Part model, mm, in its own coordinate system. Face numbers are marked on the shaded views. A direction names the side the tool comes from. Coordinates: 2 decimals unless noted, no trailing zeros. Write each loop counter-clockwise with the first axis right and the second up, starting at its lowest first coordinate (ties: lowest second). Pieces come first, ordered by that corner, then holes. Notation, with made-up numbers: (-39, -35.5) -> (-12, -35.5) arc R3 ccw to (-12, -30.5) -> close; hole circle Ø8 at (18.25, -38.75). An arc over 180 degrees is marked (long way). Write item = value, one per line.
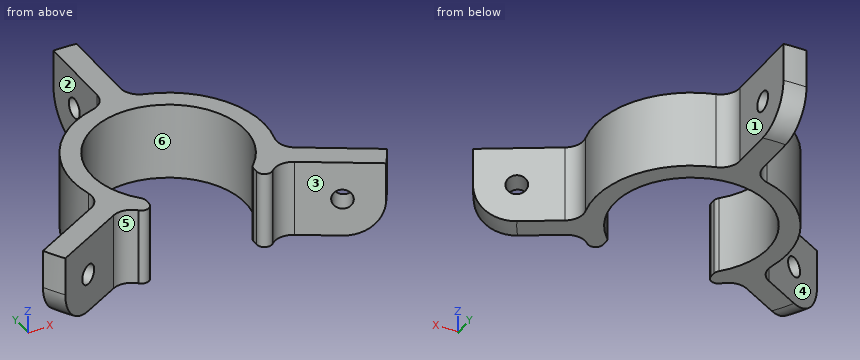
from build123d import *

# Parameters (mm, degrees)
SKETCH_R              = 50
SKETCH_R_2            = 20
PAD_DEPTH             = 20
POCKET_DEPTH          = 305.658137
POLARPATTERN_COUNT    = 3
SKETCH002_W           = 28
SKETCH002_H           = 22.742476
POCKET001_DEPTH       = 20.001
SKETCH003_R           = 2.6
POCKET002_DEPTH       = 287.850495
POLARPATTERN001_COUNT = 3
FILLET_R              = 2
FILLET001_R           = 5
FILLET002_R           = 10


with BuildPart() as part:
    # Sketch → Pad (new body)
    with BuildSketch(Plane.XY):
        Circle(SKETCH_R)
        Circle(SKETCH_R_2, mode=Mode.SUBTRACT)
    extrude(amount=PAD_DEPTH)

    # Sketch001 (on Face4 of Pad) → Pocket (cut, through all)
    with BuildSketch(Plane.XY.offset(20)):
        with BuildLine():
            ThreePointArc((22.994185, -9.811597), (21.650635, 12.5), (3, 24.819347))
            Line((3, 55.952225), (3, 24.819347))
            ThreePointArc((49.956048, -25.378036), (48.525649, 28.016297), (3, 55.952225))
            Line((22.994185, -9.811597), (49.956048, -25.378036))
        make_face()
    pocket = extrude(amount=-POCKET_DEPTH, mode=Mode.SUBTRACT)

    # PolarPattern: Pocket ×3 about axis
    polarpattern_axis = Axis((0, 0, 20), (0, 0, 1))
    for i in range(1, POLARPATTERN_COUNT):
        add(pocket.rotate(polarpattern_axis, i * 360 / POLARPATTERN_COUNT), mode=Mode.SUBTRACT)

    # Sketch002 (on Face4 of PolarPattern) → Pocket001 (cut, through all)
    with BuildSketch(Plane.XY.offset(20)):
        with Locations((0, -23.477223)):
            Rectangle(SKETCH002_W, SKETCH002_H)
    extrude(amount=-POCKET001_DEPTH, mode=Mode.SUBTRACT)

    # Sketch003 (on Face5 of Pocket001) → Pocket002 (cut, through all)
    with BuildSketch(Plane.YZ.offset(3)):
        with Locations((39.909919, 10)):
            Circle(SKETCH003_R)
    pocket002 = extrude(amount=-POCKET002_DEPTH, mode=Mode.SUBTRACT)

    # PolarPattern001: Pocket002 ×3 about axis
    polarpattern001_axis = Axis((0, 0, 0), (0, 0, 1))
    for i in range(1, POLARPATTERN001_COUNT):
        add(pocket002.rotate(polarpattern001_axis, i * 360 / POLARPATTERN001_COUNT), mode=Mode.SUBTRACT)

    # Fillet
    fillet_edges = [part.edges().sort_by_distance(p)[0] for p in [
        (-14, -20.712315, 10),
        (14, -20.712315, 10),
        (14, -14.282857, 10),
        (-14, -14.282857, 10),
    ]]
    fillet(fillet_edges, radius=FILLET_R)

    # Fillet001
    fillet001_edges = [part.edges().sort_by_distance(p)[0] for p in [
        (3, 24.819347, 10),
        (22.994185, -9.811597, 10),
        (-3, 24.819347, 10),
        (-22.994185, -9.811597, 10),
        (-19.994185, -15.00775, 10),
        (19.994185, -15.00775, 10),
    ]]
    fillet(fillet001_edges, radius=FILLET001_R)

    # Fillet002
    fillet002_edges = [part.edges().sort_by_distance(p)[0] for p in [
        (43.30127, -25, 0),
        (-43.30127, -25, 0),
        (0, 50, 0),
    ]]
    fillet(fillet002_edges, radius=FILLET002_R)


solid = part.part
Q1. Pin check, flat tips, straight feed: pin 1 (10 mm diameter, centred on x = 26.5, z = 7, fed in from +Y); pin 2 (10 mm diameter, centred on x = -17, z = 11, fed in from +Y); pin 3 (5 mm diameter, centred on x = -2, z = 13.5, fed in from -Y). Stop position of each tip, or through.
Model answer:
pin_1 = 12.76
pin_2 = 21.93
pin_3 = 19.49
Q2. Saw through at D-D on z = 3.5. Give the cut face in (x, y), and give its area (3 significant figures).
Model answer:
outline = (-42.64, -21.15) arc R47.6 ccw to (-39.64, -26.35) -> (-23.54, -17.05) arc R5 cw to (-17.53, -17.82) arc R25 ccw to (-17.39, -17.96) arc R2 ccw to (-14, -16.52) -> (-14, -15.1) arc R2 ccw to (-14.55, -13.73) arc R20 cw (long way) to (14.55, -13.73) arc R2 ccw to (14, -15.1) -> (14, -16.52) arc R2 ccw to (17.39, -17.96) arc R25 ccw to (17.53, -17.82) arc R5 cw to (23.54, -17.05) -> (39.64, -26.35) arc R47.6 ccw to (42.64, -21.15) -> (26.54, -11.86) arc R5 cw to (24.2, -6.27) arc R25 ccw to (6.67, 24.09) arc R5 cw to (3, 28.91) -> (3, 47.5) arc R47.6 ccw to (-3, 47.5) -> (-3, 28.91) arc R5 cw to (-6.67, 24.09) arc R25 ccw to (-24.2, -6.27) arc R5 cw to (-26.54, -11.86) -> close
area = 973 mm²
Q3. Saw through at C-C on x = 0. Give the cut face in (y, z).
Model answer:
outline = (20, 0) -> (40, 0) arc R10 ccw to (50, 10) -> (50, 20) -> (20, 20) -> close; hole circle Ø5.2 at (39.91, 10)
Q4. Which spindle directions (+Z, -Z, +X, -X, +Y, -Y) get a long thin tool onto all of the face, cutting with end or side? Do the marked faces 1, 2 and 3. Say none if no direction does.
Model answer:
face_1 = +Z, -Z, +X, +Y
face_2 = +Z, -Z, -X, +Y
face_3 = +Z, -Z, -Y
Q5. Saw through at B-B on y = 0. Give the cut face in (x, z), and give its area (3 significant figures).
Model answer:
outline = (-25, 0) -> (-20, 0) -> (-20, 20) -> (-25, 20) -> close; (20, 0) -> (25, 0) -> (25, 20) -> (20, 20) -> close
area = 200 mm²
Q6. Saw through at A-A on x = 18.5. Give the cut face in (y, z), and give its area (3 significant figures).
Model answer:
outline = (-17.08, 0) -> (-7.6, 0) -> (-7.6, 20) -> (-17.08, 20) -> close; (7.6, 0) -> (16.82, 0) -> (16.82, 20) -> (7.6, 20) -> close
area = 374 mm²
Q7. Probe line 1 (X direction, y = 0, z = 4.75); line 2 (X direction, y = 36, z = 16); line 3 (X direction, y = -8, z = 13). List the from-to ranges inside material, lowest first. Write a range as from..to.
Model answer:
line_1 = -25..-20, 20..25
line_2 = -3..3
line_3 = -24.06..-18.33, 18.33..24.06
Q8. Mould opens along Y. For the marked faces 4, 5 and 6 say: released by +Y, released by -Y, zero draft, split by the parting line, or undercut.
Model answer:
face_4 = released by +Y
face_5 = released by -Y
face_6 = undercut
